from build123d import *

# Parameters (mm, degrees)
SKETCH005_R                               = 22
SKETCH005_R_2                             = 12
SKETCH005_R_3                             = 2
EXTRUDE005_DEPTH                          = 10
SKETCH004_AS_DRAWN_R                      = 3.2
SKETCH004_AS_DRAWN_W                      = 12
SKETCH004_AS_DRAWN_H                      = 8
EXTRUDE004_DEPTH                          = 5
EXTRUDE004_ONTO_SKETCH004_ROLL_ANGLE      = 90
EXTRUDE004_ONTO_SKETCH004_PLACEMENT_ANGLE = 180
EXTRUDE003_DEPTH                          = 3
SKETCH002_W                               = 11
SKETCH002_H                               = 8
EXTRUDE002_DEPTH                          = 5
SKETCH_AS_DRAWN_W                         = 18
SKETCH_AS_DRAWN_H                         = 10
EXTRUDE_DEPTH                             = 5
EXTRUDE_ONTO_SKETCH_ROLL_ANGLE            = 90
SKETCH001_R                               = 4
SKETCH001_R_2                             = 1.4
SKETCH001_R_3                             = 2.75
EXTRUDE001_DEPTH                          = 25
BOX001_W                                  = 116
BOX001_H                                  = 107
BOX001_DEPTH                              = 40
BOX_W                                     = 120
BOX_H                                     = 111
BOX_DEPTH                                 = 40
FILLET_R                                  = 3
CHAMFER_SIZE                              = 1


with BuildPart() as extrude_lite:
    # Sketch005 → Extrude005 (new body)
    with BuildSketch(Plane.XY.offset(2)):
        Circle(SKETCH005_R)
        with Locations((-37, -29)):
            Circle(SKETCH005_R_2)
        with Locations((37, -29)):
            Circle(SKETCH005_R_2)
        with Locations((-44, 30)):
            Circle(SKETCH005_R_3)
        with Locations((-35, 30)):
            Circle(SKETCH005_R_3)
        with Locations((-26, 30)):
            Circle(SKETCH005_R_3)
        with Locations((-26, 20)):
            Circle(SKETCH005_R_3)
        with Locations((-35, 20)):
            Circle(SKETCH005_R_3)
        with Locations((-44, 20)):
            Circle(SKETCH005_R_3)
        with Locations((-44, 10)):
            Circle(SKETCH005_R_3)
        with Locations((-35, 10)):
            Circle(SKETCH005_R_3)
        with Locations((-26, 10)):
            Circle(SKETCH005_R_3)
        with Locations((-44, 0)):
            Circle(SKETCH005_R_3)
        with Locations((-35, 0)):
            Circle(SKETCH005_R_3)
        with Locations((-26, 0)):
            Circle(SKETCH005_R_3)
        with Locations((26, 0)):
            Circle(SKETCH005_R_3)
        with Locations((35, 0)):
            Circle(SKETCH005_R_3)
        with Locations((44, 0)):
            Circle(SKETCH005_R_3)
        with Locations((44, 10)):
            Circle(SKETCH005_R_3)
        with Locations((44, 20)):
            Circle(SKETCH005_R_3)
        with Locations((44, 30)):
            Circle(SKETCH005_R_3)
        with Locations((35, 30)):
            Circle(SKETCH005_R_3)
        with Locations((26, 30)):
            Circle(SKETCH005_R_3)
        with Locations((26, 20)):
            Circle(SKETCH005_R_3)
        with Locations((35, 20)):
            Circle(SKETCH005_R_3)
        with Locations((35, 10)):
            Circle(SKETCH005_R_3)
        with Locations((26, 10)):
            Circle(SKETCH005_R_3)
    extrude(amount=-EXTRUDE005_DEPTH)


with BuildPart() as extrude_antenna:
    # Sketch004 as drawn → Extrude004 (new)
    with BuildSketch(Plane.XY):
        with Locations((-25, 10)):
            Circle(SKETCH004_AS_DRAWN_R)
        with Locations((-35, 24.5)):
            Rectangle(SKETCH004_AS_DRAWN_W, SKETCH004_AS_DRAWN_H)
        with Locations((41, 24.5)):
            Rectangle(SKETCH004_AS_DRAWN_W, SKETCH004_AS_DRAWN_H)
    extrude(amount=-EXTRUDE004_DEPTH)


with BuildPart() as extrude_antenna_1:
    # Extrude004 onto Sketch004 roll: moved
    add(extrude_antenna.part.rotate(Axis((0, 0, 0), (1, 0, 0)), EXTRUDE004_ONTO_SKETCH004_ROLL_ANGLE))


with BuildPart() as extrude_antenna_2:
    # Extrude004 onto Sketch004 placement: moved
    add(extrude_antenna_1.part.moved(Location((0, 55, 0))).rotate(Axis((0, 55, 0), (0, 0, 1)), EXTRUDE004_ONTO_SKETCH004_PLACEMENT_ANGLE))


with BuildPart() as extrude_pwm:
    # Sketch003 → Extrude003 (new body)
    with BuildSketch(Plane(origin=(-62, 0, 0), x_dir=(0, -1, 0), z_dir=(-1, 0, 0))):
        Polygon((-34, 30), (45, 30), (45, 18), (-14, 18), (-14, 13), (-34, 13), align=None)
    extrude(amount=-EXTRUDE003_DEPTH)


with BuildPart() as extrude_wall_plug:
    # Sketch002 → Extrude002 (new body)
    with BuildSketch(Plane.YZ.offset(58)):
        Polygon((-25.5, 30), (13.5, 30), (13.5, 17), (-14.5, 17), (-14.5, 14), (-25.5, 14), align=None)
        with Locations((31, 26)):
            Rectangle(SKETCH002_W, SKETCH002_H)
    extrude(amount=-EXTRUDE002_DEPTH)


with BuildPart() as extrude_battery:
    # Sketch as drawn → Extrude (new)
    with BuildSketch(Plane.XY):
        with Locations((11, 7)):
            Rectangle(SKETCH_AS_DRAWN_W, SKETCH_AS_DRAWN_H)
        with Locations((-36, 7)):
            Rectangle(SKETCH_AS_DRAWN_W, SKETCH_AS_DRAWN_H)
    extrude(amount=-EXTRUDE_DEPTH)


with BuildPart() as extrude_battery_1:
    # Extrude onto Sketch roll: moved
    add(extrude_battery.part.rotate(Axis((0, 0, 0), (1, 0, 0)), EXTRUDE_ONTO_SKETCH_ROLL_ANGLE))


with BuildPart() as extrude_battery_2:
    # Extrude onto Sketch placement: moved
    add(extrude_battery_1.part.moved(Location((0, -56, 0))))


with BuildPart() as mount_extrude:
    # Sketch001 → Extrude001 (new body)
    with BuildSketch(Plane.XY.offset(2)):
        with Locations((-50.25, -47.25)):
            Circle(SKETCH001_R)
        with Locations((-50.25, -47.25)):
            Circle(SKETCH001_R_2, mode=Mode.SUBTRACT)
        with Locations((50.25, 47.25)):
            Circle(SKETCH001_R)
        with Locations((50.25, 47.25)):
            Circle(SKETCH001_R_2, mode=Mode.SUBTRACT)
        with Locations((-50.25, 47.25)):
            Circle(SKETCH001_R)
        with Locations((-50.25, 47.25)):
            Circle(SKETCH001_R_2, mode=Mode.SUBTRACT)
        with Locations((25.25, -42.25)):
            Circle(SKETCH001_R)
        with Locations((25.25, -42.25)):
            Circle(SKETCH001_R_2, mode=Mode.SUBTRACT)
        with Locations((51.25, -50.25)):
            Circle(SKETCH001_R_3)
        with Locations((-14.75, -39.25)):
            Circle(SKETCH001_R)
        with Locations((-14.75, -39.25)):
            Circle(SKETCH001_R_2, mode=Mode.SUBTRACT)
    extrude(amount=EXTRUDE001_DEPTH)


with BuildPart() as inner:
    # Box001 → Box001 (new body)
    with BuildSketch(Plane(origin=(-60, -54, 2), x_dir=(1, 0, 0), z_dir=(0, 0, 1))):
        with Locations((58, 53.5)):
            Rectangle(BOX001_W, BOX001_H)
    extrude(amount=BOX001_DEPTH)


with BuildPart() as chamfer_body:
    # Box → Box (new body)
    with BuildSketch(Plane(origin=(-62, -56, 0), x_dir=(1, 0, 0), z_dir=(0, 0, 1))):
        with Locations((60, 55.5)):
            Rectangle(BOX_W, BOX_H)
    extrude(amount=BOX_DEPTH)

    # Cut: cut Inner
    add(inner.part, mode=Mode.SUBTRACT)

    # Fusion: union Mount Extrude
    add(mount_extrude.part)

    # Cut001: cut Extrude Battery
    add(extrude_battery_2.part, mode=Mode.SUBTRACT)

    # Cut002: cut Extrude Wall Plug
    add(extrude_wall_plug.part, mode=Mode.SUBTRACT)

    # Cut003: cut Extrude PWM
    add(extrude_pwm.part, mode=Mode.SUBTRACT)

    # Cut004: cut Extrude Antenna
    add(extrude_antenna_2.part, mode=Mode.SUBTRACT)

    # Cut005: cut Extrude Lite
    add(extrude_lite.part, mode=Mode.SUBTRACT)

    # Fillet
    fillet_edges = [chamfer_body.edges().sort_by_distance(p)[0] for p in [
        (-62, -56, 20),
        (-62, 55, 20),
        (58, -56, 20),
        (58, 55, 20),
    ]]
    fillet(fillet_edges, radius=FILLET_R)

    # Chamfer
    chamfer_edges = [chamfer_body.edges().sort_by_distance(p)[0] for p in [
        (21.25, -42.25, 2),
        (-54.25, -47.25, 2),
        (-18.75, -39.25, 2),
        (46.25, 47.25, 2),
        (-54.25, 47.25, 2),
    ]]
    chamfer(chamfer_edges, length=CHAMFER_SIZE)


solid = chamfer_body.part
CAD build for the part. Positions are in the model's coordinates, mm. A direction names the side the tool comes from. Round coordinates to 2 decimals unless told otherwise and drop trailing zeros. Order: outer loops, then holes, each group sorted by start corner. A loop starts at its lowest first (then second) coordinate and runs counter-clockwise, first axis right, second up. Notation, with made-up numbers: (86, 38) -> (143, 38) arc R25 cw to (143, 59) -> close; hole circle Ø6 at (86, 69.5). An arc over 180 degrees is marked (long way). Write each question's results on one line, items separated by ' | '.
1. Cut at B-B (z = 24.5). Count the separate pieces of the cut face and the enclosed holes in it, plus the area to 3 significant figures.
Findings below:
separate pieces: 11 | enclosed holes: 5 | area: 839 mm²
2. Cut at A-A (x = 0). Give the cut face in (y, z), plus the area to 3 significant figures.
Findings below:
outline: (-56, 0) -> (-22, 0) -> (-22, 2) -> (-54, 2) -> (-54, 40) -> (-56, 40) -> close; (22, 0) -> (55, 0) -> (55, 40) -> (53, 40) -> (53, 2) -> (22, 2) -> close | area: 286 mm²
3. Wall check: line 1 along X through (y, z) = (18.5, 5); line 2 along Y through (x, z) = (-32, 33); line 3 along Y through (x, z) = (48, 19.5). Give the ranges that are in metal, low to high. Write a range as [from, to].
Findings below:
line 1: x = [-62, -60], [56, 58] | line 2: y = [-56, -54], [53, 55] | line 3: y = [-56, -54], [43.94, 50.56], [53, 55]
4. Pull direction X, two halves, no side cores. Call faces 1 (the face through (-3, 25, 0)), 2 (the face through (-26, 22, 1)), 3 (the face through (57.1, -55.14, 20.28)): pulls with the +X half, pulls with the -X half, needs draft (parallel to the pull), parting line crosses it, or undercut.
Findings below:
face 1: needs draft | face 2: undercut | face 3: pulls with the +X half
5. 3-axis set-ups, long thin cutter, end or side, ignore diameter. For faces 4 (the face through (-33.092, 10.601, 1.014)), 5 (the face through (-53.424, 44.816, 14.832)): which of +Z, -Z, +X, -X, +Y, -Y reach the whole face in a straight line?
Findings below:
face 4: +Z, -Z | face 5: +Z
6. Cut at C-C (y = -19). Give the cut face in (x, z).
Findings below:
outline: (-62, 0) -> (-43.63, 0) -> (-43.63, 2) -> (-60, 2) -> (-60, 18) -> (-62, 18) -> close; (-62, 30) -> (-60, 30) -> (-60, 40) -> (-62, 40) -> close; (-30.37, 0) -> (-11.09, 0) -> (-11.09, 2) -> (-30.37, 2) -> close; (11.09, 0) -> (30.37, 0) -> (30.37, 2) -> (11.09, 2) -> close; (43.63, 0) -> (58, 0) -> (58, 14) -> (56, 14) -> (56, 2) -> (43.63, 2) -> close; (56, 30) -> (58, 30) -> (58, 40) -> (56, 40) -> close
7. Flat gauge pins, fed straight in: P1, Ø10, axis at x = -25, y = 19, coming from the -Z side; P2, Ø1.4, axis at x = 24.5, y = -43, coming from the +Z side; P3, Ø1.4, axis at x = -50, y = -47.5, coming from the +Z side. Where does each tip first touch, or does it go through?
Findings below:
P1: stops at z = 0 | P2: stops at z = 27 | P3: stops at z = 2
